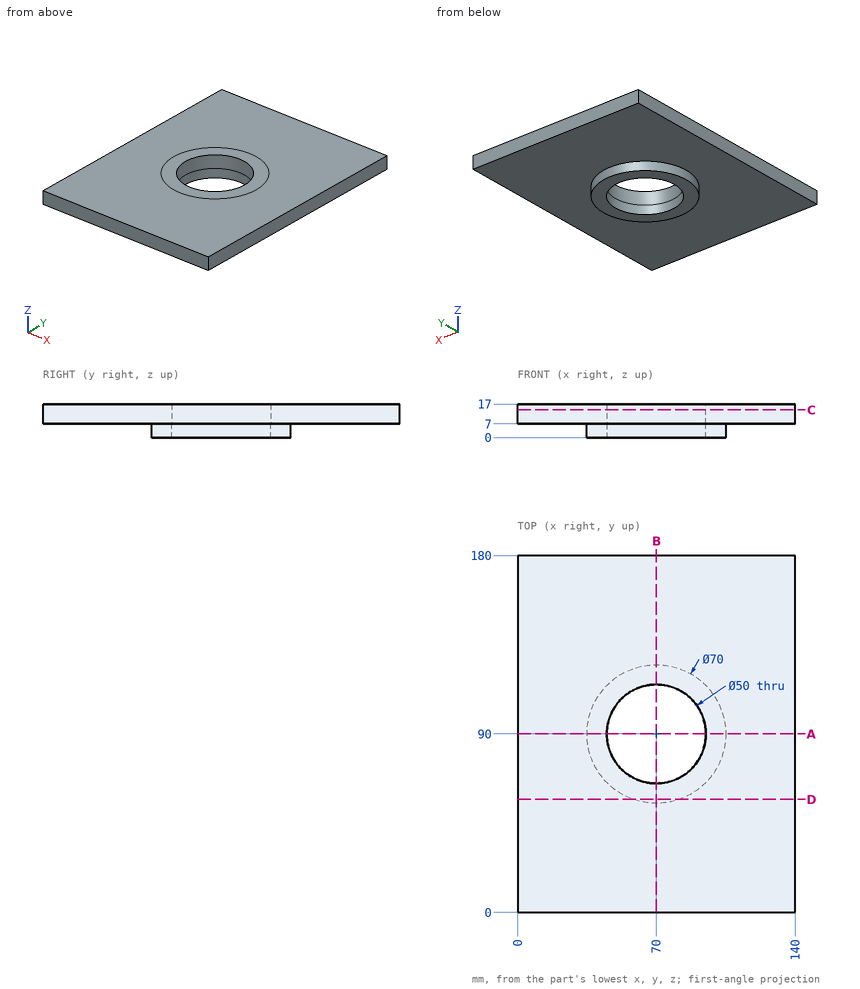
Geometry: see drawing. Coordinates: mm, zero at the bounding-box minimum. Coordinates: 2 decimals unless noted, no trailing zeros. Write each loop counter-clockwise with the first axis right and the second up, starting at its lowest first coordinate (ties: lowest second). Pieces come first, ordered by that corner, then holes. Notation, with made-up numbers: (-39, 57.25) - (-35, 57.25) arc R33 ccw to (-35, 92.25) - close; hole circle Ø1 at (-38, -36.5). An arc over 180 degrees is marked (long way). Put each result on its own line as item: value. Start each with the question number.
1) Contact query for a flat-ended pin moving along its axis: pin 1 (6 mm diameter, centred on x = 16, y = 92, fed in from -Z). Output: stop coordinate, or through.
2) Cut plane D-D (y = 57). Return the cut outline in (x, z).
3) Ray query, L1, parallel to Y at x = 70, z = 9.75; L2, parallel to Y at x = 70, z = 4; L3, parallel to X at y = 90, z = 10.75. Return the intervals inside material, ascending.
4) Cut plane C-C (z = 14). Return the cut outline in (x, y), plus the area to 3 significant figures.
5) Cut plane A-A (y = 90). Return the cut outline in (x, z), plus the area to 3 significant figures.
6) Cut plane B-B (x = 70). Return the cut outline in (y, z).
Resolved:
1. pin 1: stops at z = 7
2. outline: (0, 7) - (58.34, 7) - (58.34, 0) - (81.66, 0) - (81.66, 7) - (140, 7) - (140, 17) - (0, 17) - close
3. L1: y = 0 to 65, 115 to 180
3. L2: y = 55 to 65, 115 to 125
3. L3: x = 0 to 45, 95 to 140
4. outline: (0, 0) - (140, 0) - (140, 180) - (0, 180) - close; hole circle Ø50 at (70, 90)
4. area: 23,200 mm2
5. outline: (0, 7) - (35, 7) - (35, 0) - (45, 0) - (45, 17) - (0, 17) - close; (95, 0) - (105, 0) - (105, 7) - (140, 7) - (140, 17) - (95, 17) - close
5. area: 1,040 mm2
6. outline: (0, 7) - (55, 7) - (55, 0) - (65, 0) - (65, 17) - (0, 17) - close; (115, 0) - (125, 0) - (125, 7) - (180, 7) - (180, 17) - (115, 17) - close
